```python
from build123d import *

# Parameters (mm, degrees)
SKETCH1_W           = 34
SKETCH1_H           = 17
BOSS_EXTRUDE1_DEPTH = 4
SKETCH2_R           = 1.5
CUT_EXTRUDE1_DEPTH  = 20.4229246
SKETCH3_W           = 4.299826773
SKETCH3_H           = 10.17393153
BOSS_EXTRUDE2_DEPTH = 10


with BuildPart() as part:
    # Sketch1 → Boss-Extrude1 (new body)
    with BuildSketch(Plane(origin=(0, 0, 0), x_dir=(0, 0, -1), z_dir=(1, 0, 0))):
        Rectangle(SKETCH1_W, SKETCH1_H)
    extrude(amount=BOSS_EXTRUDE1_DEPTH)

    # Sketch2 → Cut-Extrude1 (cut, through all)
    with BuildSketch(Plane(origin=(4, 0, 0), x_dir=(0, 0, -1), z_dir=(1, 0, 0))):
        with Locations((-15.3, 6.8)):
            Circle(SKETCH2_R)
        with Locations((-15.3, -6.8)):
            Circle(SKETCH2_R)
        with Locations(Location((15.3, -6.8, 0), (0, 0, 180))):
            Circle(SKETCH2_R)
        with Locations(Location((15.3, 6.8, 0), (0, 0, 180))):
            Circle(SKETCH2_R)
    extrude(amount=-CUT_EXTRUDE1_DEPTH, mode=Mode.SUBTRACT)

    # Sketch3 → Boss-Extrude2 (add)
    with BuildSketch(Plane(origin=(4, 0, 0), x_dir=(0, 0, -1), z_dir=(1, 0, 0))):
        with Locations((8.693678476, 0)):
            Rectangle(SKETCH3_W, SKETCH3_H)
    extrude(amount=BOSS_EXTRUDE2_DEPTH)


solid = part.part
```
The model under review builds one solid part; all positions refer to its coordinate system, in mm. A direction names the side the tool comes from. Round coordinates to 2 decimals unless told otherwise and drop trailing zeros. Loops run counter-clockwise (first coordinate to the right, second up) from the corner with the lowest first, then second, coordinate; pieces in that order, holes last.
Item 1: Take a section at B-B (y = -6.8). Write out the cut boundary in (x, z).
Determined:
outline: (0, -17) - (4, -17) - (4, -16.8) - (0, -16.8) - close; (0, -13.8) - (4, -13.8) - (4, 13.8) - (0, 13.8) - close; (0, 16.8) - (4, 16.8) - (4, 17) - (0, 17) - close
Item 2: For faces 5 (the face through (9, -5.087, -9)), 6 (the face through (9, 0, -10.844)), 7 (the face through (9, 5.087, -9)), list the 3-axis set-ups (+Z, -Z, +X, -X, +Y, -Y) from which the entire face can be reached by the end or side of a thin tool; tool diameter is ignored.
Determined:
face 5: +Z, -Z, +X, -Y
face 6: -Z, +X, +Y, -Y
face 7: +Z, -Z, +X, +Y
Item 3: Take a section at D-D (x = 5). Write out the cut boundary in (y, z), then the cut area to 3 significant figures.
Determined:
outline: (-5.09, -10.84) - (5.09, -10.84) - (5.09, -6.54) - (-5.09, -6.54) - close
area: 43.7 mm2
Item 4: Clearance check with flat-ended pins moving along their axes: pin 1 Ø3.5 at (y, z) = (-6.8, 15.3) entering from +X; pin 2 Ø1 at (x, z) = (8, -6.5) entering from -Y; pin 3 Ø3 at (x, y) = (10, 4) entering from +Z. State where each tip first meets the part, or that it passes through.
Determined:
pin 1: stops at x = 4
pin 2: stops at y = -5.09
pin 3: stops at z = -6.54
Item 5: Take a section at A-A (z = 15.3). Write out the cut boundary in (x, y), then the cut area to 3 significant figures.
Determined:
outline: (0, -8.5) - (4, -8.5) - (4, -8.3) - (0, -8.3) - close; (0, -5.3) - (4, -5.3) - (4, 5.3) - (0, 5.3) - close; (0, 8.3) - (4, 8.3) - (4, 8.5) - (0, 8.5) - close
area: 44.0 mm2
Item 6: Take a section at C-C (y = 3.5). Write out the cut boundary in (x, z), then the cut area to 3 significant figures.
Determined:
outline: (0, -17) - (4, -17) - (4, -10.84) - (14, -10.84) - (14, -6.54) - (4, -6.54) - (4, 17) - (0, 17) - close
area: 179 mm2
Item 7: Mouldability with a two-part tool opening along Y and no side actions: class faces 1 (the face through (2.028, -8.264, 15.625)), 2 (the face through (2, -8.5, 0)), 3 (the face through (2.028, -8.287, -15.495)), 4 (the face through (9, 0, -6.544)) as released by +Y, released by -Y, zero draft, split by the parting line, or undercut.
Determined:
face 1: undercut
face 2: released by -Y
face 3: undercut
face 4: zero draft
Item 8: For line 1 (Y direction, x = 2.15, z = 15.3); line 2 (Z direction, x = 2.5, y = 6.25); line 3 (X direction, y = 7, z = -11), list the stretches that pass through material, from the lowest coordinate up.
Determined:
line 1: y = -8.5 to -8.3, -5.3 to 5.3, 8.3 to 8.5
line 2: z = -17 to -16.7, -13.9 to 13.9, 16.7 to 17
line 3: x = 0 to 4
